Autodesk Inventor part; units mm, degrees
ref_plane "YZ Plane" through (0, 0, 0) normal (1, 0, 0) x (0, 1, 0)
ref_plane "XZ Plane" through (0, 0, 0) normal (0, 1, 0) x (-1, 0, 0)
ref_plane "XY Plane" through (0, 0, 0) normal (0, 0, 1) x (1, 0, 0)
sketch "Эскиз1" plane through (0, 0, 0) normal (0, 0, 1) x (1, 0, 0)
  line L0 (10, 0) -> (10, 10)
  line L1 (10, 10) -> (3, 10)
  line L2 (3, 10) -> (1.8448, 9.1888)
  line L3 (1.1552, 9.1888) -> (0, 10)
  line L4 (0, 10) -> (0, 13)
  line L5 (0, 13) -> (-4, 13)
  line L6 (-4, 13) -> (-4, 10.9697)
  line L7 (-4, 10.9697) -> (-4.8, 10.9697)
  line L8 (-4.8, 10.9697) -> (-4.8, 0)
  line L9 (-4.8, 0) -> (10, 0)
  arc A0 (1.1552, 9.1888) -> (1.8448, 9.1888) centre (1.5, 9.6798) ccw
  line L10 (-7.8876, 0) -> (13.7255, 0)
  line L11 (0, -2.6) -> (0, 15.6)
  line L12 (2.3733, 9.0798) -> (10.6379, 9.0798) construction
  dimension "d0" = 0.6
  dimension "d1" = 20
  dimension "d2" = 26
  dimension "d3" = 10
  dimension "d4" = 3
  dimension "d5" = 1.5
  dimension "d6" = 21.9393
  dimension "d7" = 4
  dimension "d8" = 0.8
  dimension "d10" = 18.1596
revolve "Базовый элемент" add sketch "Эскиз1" angle 360 about axis through (-4.8, 0, 0) along (1, 0, 0)
sketch "Эскиз2" plane through (-4.8, 0, 0) normal (-1, 0, 0) x (0, 0, 1)
  circle A0 centre (0, 0) radius 10.9697
  line L0 (10.9697, 0) -> (5.4848, -9.5)
  line L1 (5.4848, -9.5) -> (-5.4848, -9.5)
  line L2 (-5.4848, -9.5) -> (-10.9697, 0)
  line L3 (-10.9697, 0) -> (-5.4848, 9.5)
  line L4 (-5.4848, 9.5) -> (5.4848, 9.5)
  line L5 (5.4848, 9.5) -> (10.9697, 0)
extrude "С головкой" add sketch "Эскиз2" along normal blind 7 contours L0 L1 L2 L3 L4 L5
fillet "Сопряжение1" radius 1 1 edges at (-4, -13, 0)
sketch "Эскиз3" plane through (0, 0, 0) normal (0, 1, 0) x (-1, 0, 0)
  line L0 (10.75, 10.9697) -> (11.8, 9.151)
  line L1 (11.8, 9.151) -> (11.8, 10.9697)
  line L2 (11.8, 10.9697) -> (10.75, 10.9697)
  line L3 (12.01, 0) -> (10.54, 0)
  dimension "d14" = 1.05
  dimension "d15" = 30
revolve "Фаска1" cut sketch "Эскиз3" angle 360 about axis through (-10, 0, 0) along (1, 0, 0)
thread "Резьба1"
chamfer "Фаска2" distance 0.9202 distance2 0.9202 1 edges at (10, -10, 0) measured on face at (7.6667, 9.9676, -0.8047)
sketch "Эскиз4" plane through (10, 0, 0) normal (1, 0, 0) x (0, 0, -1)
  point P0 (0, 0)
  point P1 (0, 0)
  point P2 (-18.5467, -33.5081)
hole "Отверстие1" at (10, 0, 0) at (10, -33.5081, 18.5467) direction (-1, 0, 0) diameter 8 depth 18 tip angle 118
sketch "Эскиз5" plane through (0, 0, 0) normal (0, 1, 0) x (-1, 0, 0)
  line L0 (-14.4667, 0) -> (16.8, 0) construction
  line L1 (0, -18.2) -> (0, 18.2) construction
  circle A0 centre (8, 0) radius 1.5
  point P0 (0, 0)
  dimension "d32" = 3
  dimension "d33" = 8
extrude "Выдавливание2" cut sketch "Эскиз5" along normal through all both and the other way through all
extrude "Выдавливание3" add sketch "Эскиз5" along normal mid plane 10
chamfer "Фаска3" distance 0.5 angle 45 2 edges at (-6.5, -9.5, 0) (-6.5, 9.5, 0)
equation "\"d12\" = KOH"
equation "\"d14\" = 0.15 * KOH"
equation "\"d17\" = RR"
equation "\"d20\" = NLG"
equation "\"d18\" = GAL"
equation "\"d19\" = -0.5 * GD1 + 0.5 * NND"
equation "\"d0\" = 0.2 * GAL1"
equation "\"d1\" = NND"
equation "\"d2\" = KOD"
equation "\"d3\" = NLG"
equation "\"d4\" = GAL1"
equation "\"d5\" = 0.5 * GAL1"
equation "\"d6\" = n_D"
equation "\"d7\" = SD"
equation "\"d8\" = PHH"
equation "\"d10\" = GD1"
equation "\"NLG\" = 10"
equation "\"NND\" = 20"
equation "\"SD\" = 4"
equation "\"PHH\" = 0.8"
equation "\"SW\" = 19"
equation "\"GAL1\" = 3"
equation "\"KOH\" = 7"
equation "\"KOD\" = 26"
equation "\"GAL\" = 0.61345 * PTC"
equation "\"RR\" = 1"
equation "\"GD1\" = THREADDIA - 1.2269 * PTC"
equation "\"n_D\" = 1.1547 * SW"
equation "\"GUL\" = 0.61345 * PTC"
equation "\"TOA\" = 30deg"
equation "\"PTC\" = 1.5"
properties part number "CSN 02 1915.21 - M 20 x 10" material "Сталь, мягкая"
Source: CAD feature listing. Evaluate the final solid. Frame: model axes, mm. A direction names the side the tool comes from. Coordinates: 2 decimals unless noted, no trailing zeros. Loops run counter-clockwise (first coordinate to the right, second up) from the corner with the lowest first, then second, coordinate; pieces in that order, holes last. Notation, with made-up numbers: (13.5, 24.5) -> (47.5, 24.5) arc R29 ccw to (47.5, 51.5) -> close; hole circle Ø2 at (83, 14.25). An arc over 180 degrees is marked (long way). Answer in a Markdown table with one row per item. Add a question column.
Q1. Pull-direction query (X, two-part tool) for faces 1 (the face through (-4.8, -10, 0)), 2 (the face through (0.874, 1.532, -3.695)), 3 (the face through (-8, -5, 0)); classes: pulls with the +X half, pulls with the -X half, needs draft (parallel to the pull), parting line crosses it, or undercut.
Q2. Contact query for flat-ended pins moving along their axis: pin 1 Ø1.6 at (y, z) = (-7, -8.5) entering from -X; pin 2 Ø7.5 at (x, z) = (-8, 1) entering from -Y; pin 3 Ø3 at (x, z) = (-5, 8.5) entering from +Y. Output: stop coordinate, or through.
Q3. Section A-A on x = -2.25. Return the cut outline in (y, z).
Q4. Ray query, line 1 along Z through (x, y) = (-7.25, -0.5); line 2 along X through (y, z) = (6.5, 0); line 3 along Z through (x, y) = (6.5, -0.25). Return the intervals inside material, ascending.
Q5. Section B-B on x = 0.75. Return the cut outline in (y, z), and give its area (3 significant figures).
Q6. Reachability of faces 4 (the face through (-4.41, -2.38, 10.71)), 5 (the face through (-9.986, 0.586, -0.373)), 6 (the face through (-4.8, 5, -9)), 7 (the face through (-8.2, -4.8, -8.2)), 8 (the face through (-8, 5, 0)) from +Z, -Z, +X, -X, +Y, -Y: full face, straight path, thin tool, end or side. Return the list, or none.
Computed values:
| question | item | result |
|---|---|---|
| 1 | face 1 | pulls with the -X half |
| 1 | face 2 | needs draft |
| 1 | face 3 | undercut |
| 2 | pin 1 | stops at x = -4.8 |
| 2 | pin 2 | stops at y = -10.97 |
| 2 | pin 3 | stops at y = 10.08 |
| 3 | outline | circle Ø26 at (0, 0); hole circle Ø8 at (0, 0) |
| 4 | line 1 | z = -10.68 to -3.97, -1.3 to 1.3, 3.97 to 10.68 |
| 4 | line 2 | x = -11.8 to -9.5, -6.5 to 10 |
| 4 | line 3 | z = -10 to -3.99, 3.99 to 10 |
| 5 | outline | circle Ø18.95 at (0, 0); hole circle Ø8 at (0, 0) |
| 5 | area | 232 mm^2 |
| 6 | face 4 | -X |
| 6 | face 5 | none |
| 6 | face 6 | -Z, -X, +Y |
| 6 | face 7 | -Z, -X, -Y |
| 6 | face 8 | +Y |
